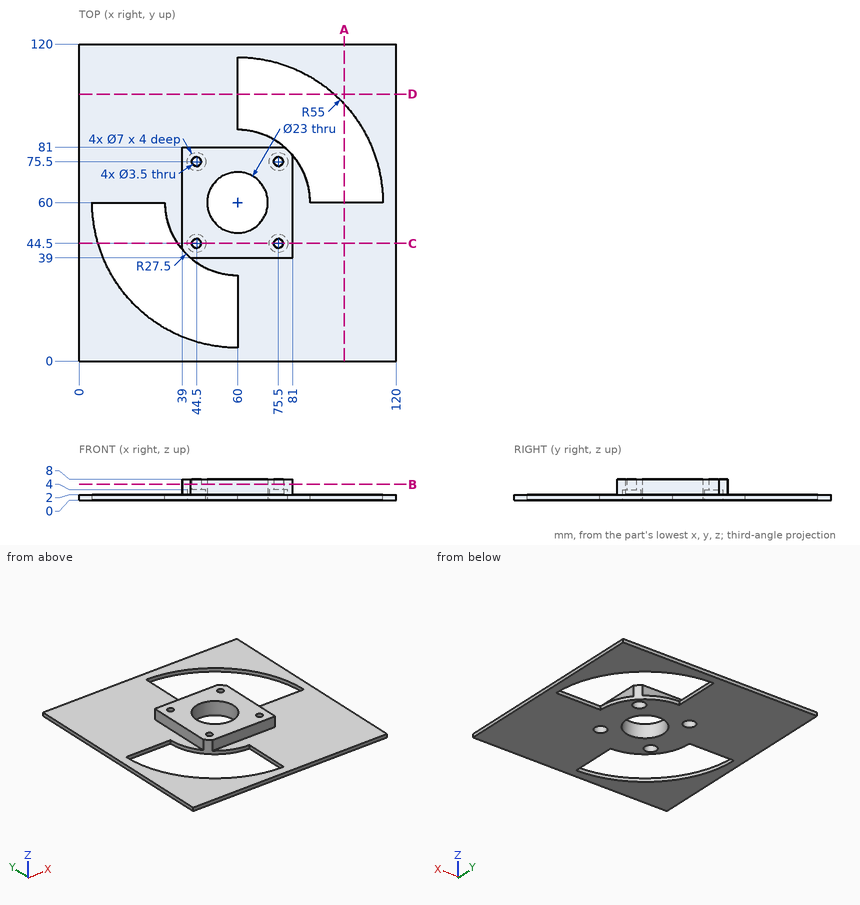
Source: three-view drawing plus pictorial views. Frame: mm from the lowest corner of the part. Give positions to 0.01 mm unless a question says otherwise; leave off trailing zeros. Write each loop counter-clockwise with the first axis right and the second up, starting at its lowest first coordinate (ties: lowest second). Pieces come first, ordered by that corner, then holes. Notation, with made-up numbers: M 63,83.5 L 113,83.5 A18 cw 113,111.5 Z; hole C 71.25,23 d11. An arc over 180 degrees is marked long. Use one line per item in the form item = value.
1. Ray query, L1, parallel to Y at x = 44.5, z = 6.6; L2, parallel to Y at x = 44.5, z = 3.15. Return the intervals inside material, ascending.
Outcome:
L1 = 39 to 42.75, 46.25 to 73.75, 77.25 to 81
L2 = 39 to 41, 48 to 72, 79 to 81
2. Cut plane A-A on x = 100.5. Return loops of the section in (y, z), and give its area (3 significant figures).
Outcome:
outline = M 0,0 L 60,0 L 60,2 L 0,2 Z; M 97.21,0 L 120,0 L 120,2 L 97.21,2 Z
area = 166 mm²
3. First-contact query: P1, Ø5.5, axis at x = 77, y = 74.5, coming from the -Z side; P2, Ø2, axis at x = 44.5, y = 75.5, coming from the +Z side; P3, Ø1.5, axis at y = 47.5, z = 3, coming from the -X side; P4, Ø5.5, axis at x = 44.5, y = 44.5, coming from the -Z side. Flat tips, straight axial feed; report the tip coordinate or a pass-through.
Outcome:
P1 = 0
P2 = through
P3 = 39
P4 = 4
4. Cut plane B-B on z = 6. Return loops of the section in (x, y), and give its area (3 significant figures).
Outcome:
outline = M 39,42.24 A27.5 ccw 42.24,39 L 81,39 L 81,77.76 A27.5 ccw 77.76,81 L 39,81 Z; hole C 44.5,44.5 d3.5; hole C 44.5,75.5 d3.5; hole C 60,60 d23; hole C 75.5,44.5 d3.5; hole C 75.5,75.5 d3.5
area = 1,300 mm²
5. Cut plane C-C on y = 44.5. Return loops of the section in (x, z).
Outcome:
outline = M 0,0 L 7.23,0 L 7.23,2 L 0,2 Z; M 37.28,0 L 41,0 L 41,4 L 42.75,4 L 42.75,8 L 39,8 L 39,2 L 37.28,2 Z; M 46.25,4 L 48,4 L 48,0 L 72,0 L 72,4 L 73.75,4 L 73.75,8 L 46.25,8 Z; M 77.25,4 L 79,4 L 79,0 L 120,0 L 120,2 L 81,2 L 81,8 L 77.25,8 Z
6. Cut plane D-D on y = 101. Return loops of the section in (x, z).
Outcome:
outline = M 0,0 L 60,0 L 60,2 L 0,2 Z; M 96.66,0 L 120,0 L 120,2 L 96.66,2 Z
